Build history of the part. All positions in model axes, mm. Face numbers are marked on the shaded views. A direction names the side the tool comes from. Give positions to 0.01 mm unless a question says otherwise; leave off trailing zeros. Write each loop counter-clockwise with the first axis right and the second up, starting at its lowest first coordinate (ties: lowest second). Pieces come first, ordered by that corner, then holes. Notation, with made-up numbers: (-12.75, 59.5) -> (39.25, 59.5) arc R26 ccw to (39.25, 91.5) -> close; hole circle Ø3 at (55.5, 50). An arc over 180 degrees is marked (long way). Write item = value, one per line. Start each with the question number.
Q1. Saw through at A-A, the plane z = 4. List the corners of the cut face in (x, y), then the cut area to 3 significant figures.
Q2. Saw through at C-C, the plane x = 5. List the corners of the cut face in (y, z), then the cut area to 3 significant figures.
Q3. Saw through at D-D, the plane x = 40. List the corners of the cut face in (y, z), then the cut area to 3 significant figures.
Q4. Mould opens along X. For the marked faces 1, 2 and 3 say: pulls with the +X half, pulls with the -X half, needs draft (parallel to the pull), parting line crosses it, or undercut.
Q5. Tool access for the marked faces 4, 5 and 6: list every direction of +Z, -Z, +X, -X, +Y, -Y with a clear straight run to the whole face (end or side of a thin tool).
Q6. Drop flat-ended pins along their axis: P1, Ø4, axis at x = 3.5, z = 2.5, coming from the -Y side; P2, Ø2, axis at y = 10, z = -0.5, coming from the -X side; P3, Ø5, axis at x = 28, z = -1, coming from the +Y side. Give the stop position or say it passes through.
Q7. Saw through at B-B, the plane y = -41.5. List the corners of the cut face in (x, z).
Q8. Wall check: line 1 (X direction, y = -2, z = 2.5); line 2 (X direction, y = 11, z = 2.75) (1 decimal); line 3 (X direction, y = -5, z = 1.5). Give the ranges that are in metal, low to high.
Autodesk Fusion 360 part; units mm, degrees
sketch "Sketch1" plane through (0, 0, 0) normal (0, 0, 1) x (1, 0, 0)
  line L0 (-65, 0) -> (67.0686, 0)
  line L1 (-35, 0) -> (-35, -80)
  line L2 (-50, 0) -> (-50, -80)
  line L3 (35, 0) -> (35, -80)
  line L4 (50, 0) -> (50, -80)
  line L5 (35, -80) -> (50, -80)
  line L6 (-50, -80) -> (-35, -80)
  arc A0 (35, 0) -> (-35, 0) centre (0, 0) ccw
  arc A1 (50, 0) -> (-50, 0) centre (0, 0) ccw
  arc A2 (38.5, 0) -> (-38.5, 0) centre (0, 0) ccw
  arc A3 (46.5, 0) -> (-46.5, 0) centre (0, 0) ccw
  line L7 (-38.5, 0) -> (-38.5, -80)
  line L8 (-46.5, 0) -> (-46.5, -80)
  line L9 (38.5, 0) -> (38.5, -80)
  line L10 (46.5, 0) -> (46.5, -80)
  dimension "d1" = 70
  dimension "d2" = 100
  dimension "d3" = 80
  dimension "d4" = 80
  dimension "d5" = 80
  dimension "d8" = 77
  dimension "d9" = 93
extrude "Extrude2" add sketch "Sketch1" along normal blind 6 contours L0 A1 A3 | L0 L2 L6 L8 | L0 L4 L5 L10 | L0 A0 A2 | L0 L1 L6 L7 | L0 L3 L5 L9 makes body 1 at (36.1667, -53.3333, 0) makes body 2 at (-47.6667, -53.3333, 0)
extrude "Extrude3" add sketch "Sketch1" along normal blind 2 separate body contours L0 A2 A3 | L0 L6 L7 L8 | L0 L5 L9 L10 makes body 3
extrude "Extrude4" add sketch "Sketch1" against normal blind 3.3 contours L0 A1 A3 | L0 L2 L6 L8 | L0 A2 A3 | L0 L6 L7 L8 | L0 L4 L5 L10 | L0 A0 A2 | L0 L1 L6 L7 | L0 L5 L9 L10 | L0 L3 L5 L9 bodies 1 2 3
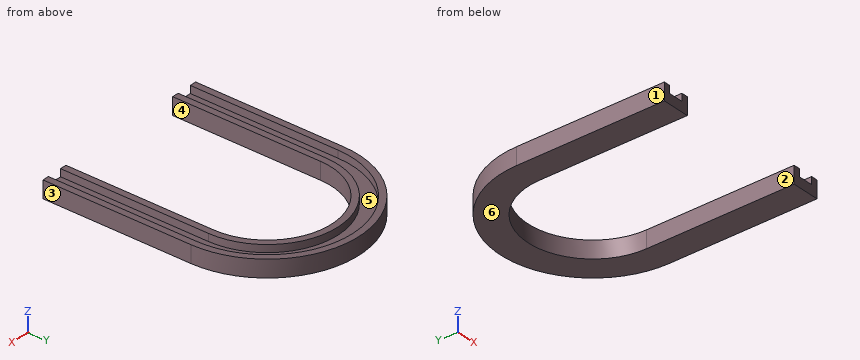
Report:
q1.outline = (-50, -80) -> (-46.5, -80) -> (-46.5, 0) arc R46.5 cw to (46.5, 0) -> (46.5, -80) -> (50, -80) -> (50, 0) arc R50 ccw to (-50, 0) -> close; (-38.5, -80) -> (-35, -80) -> (-35, 0) arc R35 cw to (35, 0) -> (35, -80) -> (38.5, -80) -> (38.5, 0) arc R38.5 ccw to (-38.5, 0) -> close
q1.area = 2,050 mm2
q2.outline = (34.64, -3.3) -> (49.75, -3.3) -> (49.75, 6) -> (46.23, 6) -> (46.23, 2) -> (38.17, 2) -> (38.17, 6) -> (34.64, 6) -> close
q2.area = 108 mm2
q3.outline = (-80, -3.3) -> (30, -3.3) -> (30, 6) -> (23.71, 6) -> (23.71, 2) -> (-80, 2) -> close
q3.area = 608 mm2
q4.face_1 = pulls with the -X half
q4.face_2 = undercut
q4.face_3 = pulls with the +X half
q5.face_4 = +Z, -Z, -Y
q5.face_5 = +Z
q5.face_6 = -Z, +X, -X, +Y, -Y
q6.P1 = 34.57
q6.P2 = -49.18
q6.P3 = 43.01
q7.outline = (-50, -3.3) -> (-35, -3.3) -> (-35, 6) -> (-38.5, 6) -> (-38.5, 2) -> (-46.5, 2) -> (-46.5, 6) -> (-50, 6) -> close; (35, -3.3) -> (50, -3.3) -> (50, 6) -> (46.5, 6) -> (46.5, 2) -> (38.5, 2) -> (38.5, 6) -> (35, 6) -> close
q8.line_1 = -50 to -46.5, -38.5 to -35, 35 to 38.5, 46.5 to 50
q8.line_2 = -48.8 to -45.2, -36.9 to -33.2, 33.2 to 36.9, 45.2 to 48.8
q8.line_3 = -50 to -35, 35 to 50
